from build123d import *

# Parameters (mm, degrees)
F0_R     = 7.5
F1_DEPTH = 25
F2_R     = 7.5
F2_R_2   = 4.95
F3_DEPTH = 20
F4_R     = 3.4
F5_DEPTH = 10
F6_R     = 0.25


with BuildPart() as f1:
    # F0 (on Top) → F1 (new body)
    with BuildSketch(Plane.XY):
        Circle(F0_R)
    extrude(amount=F1_DEPTH)

    # F2 (on face) → F3 (cut)
    with BuildSketch(Plane.XY.offset(25)):
        Circle(F2_R)
        Circle(F2_R_2, mode=Mode.SUBTRACT)
    extrude(amount=-F3_DEPTH, mode=Mode.SUBTRACT)

    # F4 (on face) → F5 (cut)
    with BuildSketch(Plane.XY.offset(25)):
        Circle(F4_R)
    extrude(amount=-F5_DEPTH, mode=Mode.SUBTRACT)

    # F6
    f6_edges = [f1.edges().sort_by_distance(p)[0] for p in [
        (-7.5, 0, 5),
        (-7.5, 0, 0),
        (-4.95, 0, 25),
        (-3.4, 0, 25),
        (-4.95, 0, 5),
    ]]
    fillet(f6_edges, radius=F6_R)


solid = f1.part
Here's how the part is built. I have some questions about the finished solid (model axes, mm). A direction names the side the tool comes from. Coordinates: 2 decimals unless noted, no trailing zeros. Write each loop counter-clockwise with the first axis right and the second up, starting at its lowest first coordinate (ties: lowest second). Pieces come first, ordered by that corner, then holes. Notation, with made-up numbers: (-5.5, 80.5) - (20.5, 80.5) arc R8 cw to (20.5, 94.5) - close; hole circle Ø5 at (77.25, 28). An arc over 180 degrees is marked (long way). Use one line per item in the form item = value.
1) I need wall thicknesses on line 1 (Y direction, x = 0, z = 17); line 2 (Z direction, x = -2.5, y = 5); line 3 (Z direction, x = 1.5, y = 3). Which ranges of each line are inside material? Lowest first, please.
Solved:
line_1 = -4.95 to -3.4, 3.4 to 4.95
line_2 = 0 to 5
line_3 = 0 to 15
2) Suppose I cut it at A-A, the plane y = 0. Write out the boundary of the cut face in (x, z).
Solved:
outline = (-7.5, 0.25) arc R0.25 ccw to (-7.25, 0) - (7.25, 0) arc R0.25 ccw to (7.5, 0.25) - (7.5, 4.75) arc R0.25 ccw to (7.25, 5) - (5.2, 5) arc R0.25 cw to (4.95, 5.25) - (4.95, 24.75) arc R0.25 ccw to (4.7, 25) - (3.65, 25) arc R0.25 ccw to (3.4, 24.75) - (3.4, 15) - (-3.4, 15) - (-3.4, 24.75) arc R0.25 ccw to (-3.65, 25) - (-4.7, 25) arc R0.25 ccw to (-4.95, 24.75) - (-4.95, 5.25) arc R0.25 cw to (-5.2, 5) - (-7.25, 5) arc R0.25 ccw to (-7.5, 4.75) - close
3) Suppose I cut it at C-C, the plane z = 20. Write out the boundary of the cut face in (x, y).
Solved:
outline = circle Ø9.9 at (0, 0); hole circle Ø6.8 at (0, 0)
4) On a 3-axis mill with a long thin cutter (end or side, diameter ignored), from which of +Z, -Z, +X, -X, +Y, -Y can I reach the whole of each face in a straight line? I mean faces 4 (the flat face through (0, -4, 25)), 5 (the cylindrical face through (4.72, 1.49, 15.14)). Say none if no direction works.
Solved:
face_4 = +Z, +X, -X, +Y, -Y
face_5 = +Z
5) Suppose I cut it at D-D, the plane z = 10.5. Write out the boundary of the cut face in (x, y), plus the area to 3 significant figures.
Solved:
outline = circle Ø9.9 at (0, 0)
area = 77.0 mm2
6) Thinking about a two-plate mould opening in X: for faces 1 (the flat face through (-2, 5, 5)), 2 (the cylindrical face through (-7.493, 0.33, 2.468)), 3 (the cylindrical face through (-0.74, -3.32, 19.94)), which applies, released by +X, released by -X, zero draft, split by the parting line, or undercut?
Solved:
face_1 = zero draft
face_2 = split by the parting line
face_3 = undercut
7) I'm going to push flat-ended pins straight in: P1, Ø3, axis at y = 2.5, z = 4.5, coming from the -X side; P2, Ø4, axis at x = 0, y = 0, coming from the +Z side; P3, Ø5, axis at y = 1.5, z = 3.5, coming from the +X side; P4, Ø4, axis at y = 4, z = 11, coming from the +X side. Where does each tip first touch, or does it pass through?
Solved:
P1 = -7.43
P2 = 15
P3 = 7.5
P4 = 4.53
